Source: CAD feature listing. Evaluate the final solid. Frame: model axes, mm. Face numbers are marked on the shaded views. A direction names the side the tool comes from. Give positions to 0.01 mm unless a question says otherwise; leave off trailing zeros. Loops run counter-clockwise (first coordinate to the right, second up) from the corner with the lowest first, then second, coordinate; pieces in that order, holes last. Notation, with made-up numbers: M -16,23 L 42,23 A17 ccw 42,32 Z; hole C 4,64 d3. An arc over 180 degrees is marked long. Answer in a Markdown table with one row per item.
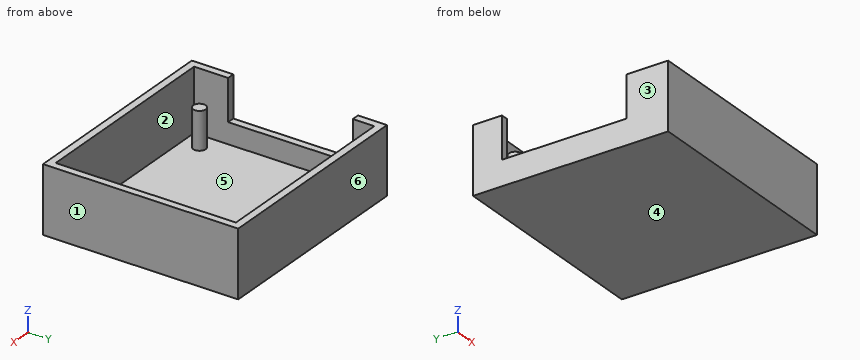
```python
from build123d import *

# Parameters (mm, degrees)
SKETCH016_W     = 52
SKETCH016_H     = 47
SKETCH016_W_2   = 48
SKETCH016_H_2   = 43
PAD006_DEPTH    = 16
SKETCH018_W     = 48
SKETCH018_H     = 43
SKETCH018_R     = 0.5
PAD007_DEPTH    = 1
SKETCH019_R     = 1.5
PAD008_DEPTH    = 10
SKETCH017_W     = 48.4
SKETCH017_H     = 43.4
SKETCH017_W_2   = 45.439167
SKETCH017_H_2   = 40.049149
POCKET005_DEPTH = 15.001
SKETCH020_W     = 2
SKETCH020_H     = 30
POCKET006_DEPTH = 10.001


with BuildPart() as part:
    # Sketch016 → Pad006 (new body)
    with BuildSketch(Plane.XY):
        with Locations((26, 23.5)):
            Rectangle(SKETCH016_W, SKETCH016_H)
        with Locations((26, 23.5)):
            Rectangle(SKETCH016_W_2, SKETCH016_H_2, mode=Mode.SUBTRACT)
    extrude(amount=PAD006_DEPTH)

    # Sketch018 → Pad007 (join)
    with BuildSketch(Plane.XY):
        with Locations((26, 23.5)):
            Rectangle(SKETCH018_W, SKETCH018_H)
        with Locations((6, 41)):
            Circle(SKETCH018_R, mode=Mode.SUBTRACT)
        with Locations((6, 6)):
            Circle(SKETCH018_R, mode=Mode.SUBTRACT)
        with Locations((46, 6)):
            Circle(SKETCH018_R, mode=Mode.SUBTRACT)
        with Locations((46, 41)):
            Circle(SKETCH018_R, mode=Mode.SUBTRACT)
    extrude(amount=PAD007_DEPTH)

    # Sketch019 → Pad008 (join)
    with BuildSketch(Plane.XY):
        with Locations((6, 41)):
            Circle(SKETCH019_R)
        with Locations((6, 6)):
            Circle(SKETCH019_R)
        with Locations((46, 6)):
            Circle(SKETCH019_R)
        with Locations((46, 41)):
            Circle(SKETCH019_R)
    extrude(amount=PAD008_DEPTH)

    # Sketch017 → Pocket005 (cut, through all)
    with BuildSketch(Plane.XY.offset(1)):
        with Locations((26, 23.5)):
            Rectangle(SKETCH017_W, SKETCH017_H)
        with Locations((26.011635, 23.557234)):
            Rectangle(SKETCH017_W_2, SKETCH017_H_2, mode=Mode.SUBTRACT)
    extrude(amount=POCKET005_DEPTH, mode=Mode.SUBTRACT)

    # Sketch020 → Pocket006 (cut, through all)
    with BuildSketch(Plane.XY.offset(6)):
        with Locations((1, 25)):
            Rectangle(SKETCH020_W, SKETCH020_H)
    extrude(amount=POCKET006_DEPTH, mode=Mode.SUBTRACT)


with BuildPart() as part_1:
    # Body003 placement: moved
    add(part.part.moved(Location((0, -47, 0))))


solid = part_1.part
```
Q1. Section query D-D (z = 10.75). Output: boundary loops of the cut face in (x, y), plus the area to 3 significant figures.
Values follow:
| item | result |
|---|---|
| outline | M 0,-47 L 52,-47 L 52,0 L 0,0 L 0,-7 L 1.8,-7 L 1.8,-1.8 L 50.2,-1.8 L 50.2,-45.2 L 1.8,-45.2 L 1.8,-37 L 0,-37 Z |
| area | 289 mm^2 |
Q2. Section query C-C (y = -34). Output: boundary loops of the cut face in (x, z).
Values follow:
| item | result |
|---|---|
| outline | M 0,0 L 52,0 L 52,16 L 50.2,16 L 50.2,1 L 1.8,1 L 1.8,6 L 0,6 Z |
Q3. Section query B-B (x = 6). Output: boundary loops of the cut face in (y, z), plus the area to 3 significant figures.
Values follow:
| item | result |
|---|---|
| outline | M -47,0 L 0,0 L 0,16 L -1.8,16 L -1.8,1 L -4.5,1 L -4.5,10 L -7.5,10 L -7.5,1 L -39.5,1 L -39.5,10 L -42.5,10 L -42.5,1 L -45.2,1 L -45.2,16 L -47,16 Z |
| area | 155 mm^2 |
Q4. Mould query, pull axis X, two halves, no side actions, for the marked faces 1, 2, 3 and 4. Classes: +X half, -X half, draft (parallel to the pull), parting line (faces both ways), or undercut.
Values follow:
| item | result |
|---|---|
| face 1 | +X half |
| face 2 | undercut |
| face 3 | -X half |
| face 4 | draft |
Q5. Reachability of the marked faces 5 and 6 from +Z, -Z, +X, -X, +Y, -Y: full face, straight path, thin tool, end or side. Return the list, or none.
Values follow:
| item | result |
|---|---|
| face 5 | +Z |
| face 6 | +Z, -Z, +X, -X, +Y |
Q6. Ray query, probe 1 along Y at (x, z) = (34, 5.5); probe 2 along X at (y, z) = (-3, 3.5); probe 3 along Y at (x, z) = (6.5, 8.25). Return the intervals inside material, ascending. Write a range as from..to.
Values follow:
| item | result |
|---|---|
| probe 1 | -47..-45.2, -1.8..0 |
| probe 2 | 0..1.8, 50.2..52 |
| probe 3 | -47..-45.2, -42.41..-39.59, -7.41..-4.59, -1.8..0 |
Q7. Section query A-A (z = 5.25). Output: boundary loops of the cut face in (x, y).
Values follow:
| item | result |
|---|---|
| outline | M 0,-47 L 52,-47 L 52,0 L 0,0 Z; C 6,-41 d3; C 6,-6 d3; C 46,-41 d3; C 46,-6 d3; hole M 1.8,-45.2 L 50.2,-45.2 L 50.2,-1.8 L 1.8,-1.8 Z |
Q8. Contact query for flat-ended pins moving along their axis: pin 1 Ø3 at (x, y) = (10, -40.5) entering from +Z; pin 2 Ø5 at (y, z) = (-20.5, 10) entering from -X; pin 3 Ø2.5 at (x, y) = (46, -41.5) entering from +Z. Output: stop coordinate, or through.
Values follow:
| item | result |
|---|---|
| pin 1 | z = 1 |
| pin 2 | x = 50.2 |
| pin 3 | z = 10 |
